Build history of the part. All positions in model axes, mm. Round coordinates to 2 decimals unless told otherwise and drop trailing zeros. Order: outer loops, then holes, each group sorted by start corner. A loop starts at its lowest first (then second) coordinate and runs counter-clockwise, first axis right, second up. Notation, with made-up numbers: (76.25, 71) -> (81.25, 71) arc R26 cw to (81.25, 98) -> close; hole circle Ø7 at (-29.75, 33.5). An arc over 180 degrees is marked (long way). Use a Markdown table: item, result. Add a question column.
Item 1: Slice it at C-C, the plane x = 60.5. Give the cut face in (y, z), plus the area to 3 significant figures.
Item 2: Probe L1, parallel to X at y = -310, z = 3; L2, parallel to X at y = 72, z = 1.8; L3, parallel to X at y = -170.5, z = 3.6. List the from-to ranges inside material, lowest first.
Item 3: Slice it at B-B, the plane y = 50.5. Give the cut face in (x, z).
Item 4: Slice it at A-A, the plane z = 3. Give the cut face in (x, y), plus the area to 3 significant figures.
Item 5: Pin check, flat tips, straight feed: pin 1 (2 mm diameter, centred on x = 62, z = 1.5, fed in from -Y); pin 2 (2 mm diameter, centred on x = 37, z = 2, fed in from +Y); pin 3 (1.8 mm diameter, centred on x = 169.17, y = -310, fed in from -Z); pin 4 (2 mm diameter, centred on y = 60, z = 2.5, fed in from -X). Stop position of each tip, or through.
from build123d import *

# Parameters (mm, degrees)
SKETCH1_W           = 31.282297403
SKETCH1_H           = 14
SKETCH1_W_2         = 31.32455923
SKETCH1_H_2         = 40
SKETCH1_W_3         = 270.751882141
SKETCH1_H_3         = 47
SKETCH1_W_4         = 200
SKETCH1_H_4         = 50
BOSS_EXTRUDE1_DEPTH = 4
SKETCH2_R           = 1.5
CUT_EXTRUDE1_DEPTH  = 451.114707602


with BuildPart() as part:
    # Sketch1 → Boss-Extrude1 (new body)
    with BuildSketch(Plane.XY):
        Polygon((25.5, 1), (25.5, -13), (25.5, -225), (25.5, -265), (65.632913627, -265), (121.5, -265), (321.5, -265), (321.5, 30), (50.748117859, 30), (25.5, 30), align=None)
        with Locations((9.858851298, -6)):
            Rectangle(SKETCH1_W, SKETCH1_H)
        with Locations((9.837720385, -245)):
            Rectangle(SKETCH1_W_2, SKETCH1_H_2)
        with Locations((186.124058929, 53.5)):
            Rectangle(SKETCH1_W_3, SKETCH1_H_3)
        with Locations((221.5, -290)):
            Rectangle(SKETCH1_W_4, SKETCH1_H_4)
    extrude(amount=BOSS_EXTRUDE1_DEPTH)

    # Sketch2 → Cut-Extrude1 (cut, through all)
    with BuildSketch(Plane(origin=(0, 0, 0), x_dir=(-1, 0, 0), z_dir=(0, 0, -1))):
        with Locations((-113.998383462, 72)):
            Circle(SKETCH2_R)
        with Locations((-88.397045893, 72)):
            Circle(SKETCH2_R)
        with Locations((-169.168895948, -310)):
            Circle(SKETCH2_R)
        with Locations((-149.084447974, -310)):
            Circle(SKETCH2_R)
    extrude(amount=-CUT_EXTRUDE1_DEPTH, mode=Mode.SUBTRACT)


solid = part.part
Check sheet entries:
| question | item | result |
|---|---|---|
| 1 | outline | (-265, 0) -> (77, 0) -> (77, 4) -> (-265, 4) -> close |
| 1 | area | 1,370 mm2 |
| 2 | L1 | 121.5 to 147.58, 150.58 to 167.67, 170.67 to 321.5 |
| 2 | L2 | 50.75 to 86.9, 89.9 to 112.5, 115.5 to 321.5 |
| 2 | L3 | 25.5 to 321.5 |
| 3 | outline | (50.75, 0) -> (321.5, 0) -> (321.5, 4) -> (50.75, 4) -> close |
| 4 | outline | (-5.82, -265) -> (121.5, -265) -> (121.5, -315) -> (321.5, -315) -> (321.5, 77) -> (50.75, 77) -> (50.75, 30) -> (25.5, 30) -> (25.5, 1) -> (-5.78, 1) -> (-5.78, -13) -> (25.5, -13) -> (25.5, -225) -> (-5.82, -225) -> close; hole circle Ø3 at (88.4, 72); hole circle Ø3 at (114, 72); hole circle Ø3 at (149.08, -310); hole circle Ø3 at (169.17, -310) |
| 4 | area | 112,000 mm2 |
| 5 | pin 1 | y = -265 |
| 5 | pin 2 | y = 30 |
| 5 | pin 3 | through |
| 5 | pin 4 | x = 50.75 |
